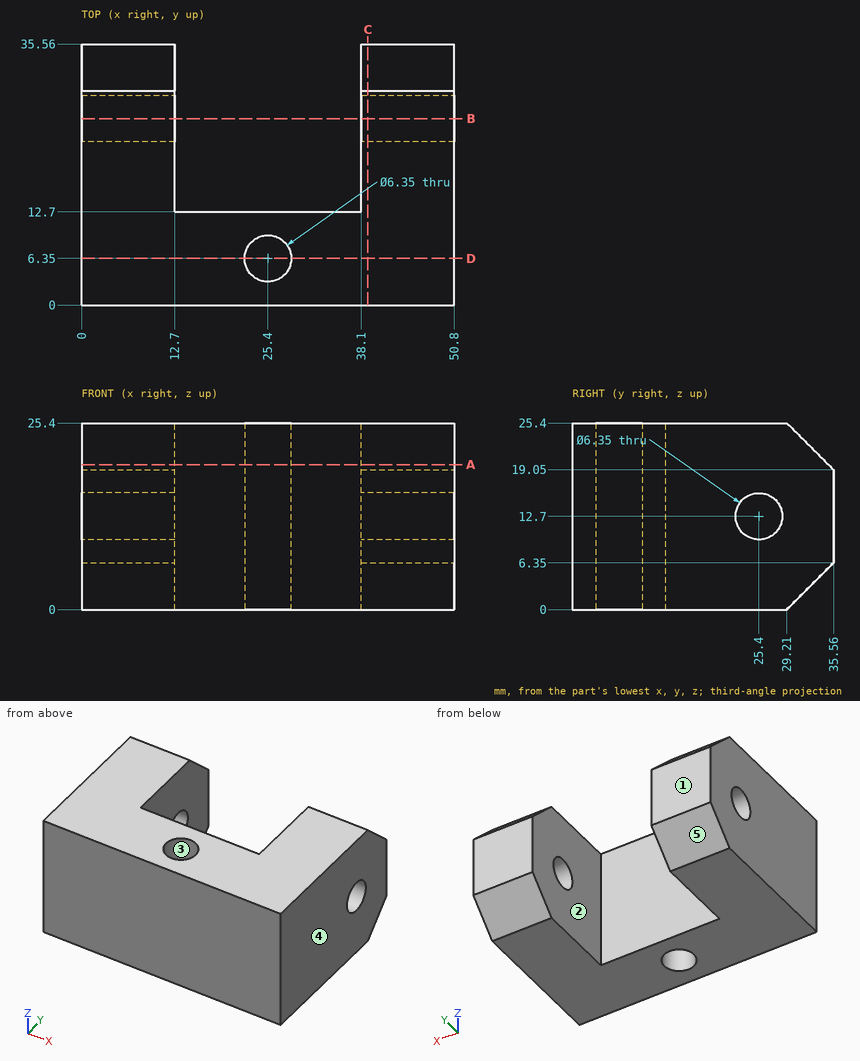
Part print with two shaded views. Sizes in mm from the minimum x, y, z corner. A direction names the side the tool comes from. Round coordinates to 2 decimals unless told otherwise and drop trailing zeros. Loops run counter-clockwise (first coordinate to the right, second up) from the corner with the lowest first, then second, coordinate; pieces in that order, holes last. Notation, with made-up numbers: M 71,8.25 L 117,8.25 A17 cw 117,28.25 Z; hole C -13.5,59.25 d6. An arc over 180 degrees is marked long. Put each result on its own line as item: value. Start each with the question number.
Item 1: Cut at B-B (y = 25.4). List the corners of the cut face in (x, z) (3 decimals).
Item 2: Drill centre lines: line 1 along X through (y, z) = (22.5, 19.75); line 2 along Y through (x, z) = (25.4, 17.25) (3 decimals); line 3 along Z through (x, y) = (8.25, 25.4) (3 decimals). Where is each one in solid material? Low to high.
Item 3: Cut at C-C (x = 39). List the corners of the cut face in (y, z) (3 decimals), then the cut area to 3 significant figures.
Item 4: Cut at D-D (y = 6.35). List the corners of the cut face in (x, z) (3 decimals), then the cut area to 3 significant figures.
Item 5: Cut at A-A (z = 19.75). List the corners of the cut face in (x, y) (3 decimals), then the cut area to 3 significant figures.
Item 6: Drop flat-ended pins along their axis: P1, Ø4, axis at y = 25.4, z = 12.7, coming from the +X side; P2, Ø1.5, axis at x = 29.5, z = 6.5, coming from the +Y side. Give the stop position or say it passes through.
Item 7: Mould opens along X. For the marked faces 3, 4 and 5 say: released by +X, released by -X, zero draft, split by the parting line, or undercut.
Item 8: 3-axis set-ups, long thin cutter, end or side, ignore diameter. For the marked faces 1 and 2: which of +Z, -Z, +X, -X, +Y, -Y reach the whole face in a straight line?
Answer block:
1. outline: M 0,0 L 12.7,0 L 12.7,9.525 L 0,9.525 Z; M 0,15.875 L 12.7,15.875 L 12.7,25.4 L 0,25.4 Z; M 38.1,0 L 50.8,0 L 50.8,9.525 L 38.1,9.525 Z; M 38.1,15.875 L 50.8,15.875 L 50.8,25.4 L 38.1,25.4 Z
2. line 1: 0 to 12.7, 38.1 to 50.8
2. line 2: 0 to 3.175, 9.525 to 12.7
2. line 3: 0 to 9.525, 15.875 to 25.4
3. outline: M 0,0 L 29.21,0 L 35.56,6.35 L 35.56,19.05 L 29.21,25.4 L 0,25.4 Z; hole C 25.4,12.7 d6.35
3. area: 831 mm2
4. outline: M 0,0 L 22.225,0 L 22.225,25.4 L 0,25.4 Z; M 28.575,0 L 50.8,0 L 50.8,25.4 L 28.575,25.4 Z
4. area: 1,130 mm2
5. outline: M 0,0 L 50.8,0 L 50.8,34.86 L 38.1,34.86 L 38.1,12.7 L 12.7,12.7 L 12.7,34.86 L 0,34.86 Z; hole C 25.4,6.35 d6.35
5. area: 1,180 mm2
6. P1: through
6. P2: y = 12.7
7. face 3: undercut
7. face 4: released by +X
7. face 5: zero draft
8. face 1: +Z, -Z, +X, -X, +Y
8. face 2: +Z, -Z, +Y
